from build123d import *

# Parameters (mm, degrees)
SKETCH_R        = 31.75
PAD_DEPTH       = 37.1475
SKETCH001_R     = 16.256
POCKET_DEPTH    = 19.9771
SKETCH002_R     = 16.256
POCKET001_DEPTH = 14.8463
PAD001_DEPTH    = 10.1219
SKETCH004_R     = 1.74625
POCKET002_DEPTH = 32.4241
SKETCH005_R     = 4.7879
POCKET003_DEPTH = 2.6924
SKETCH006_R     = 2.425304
POCKET004_DEPTH = 29.7317
SKETCH007_R     = 4.7879
POCKET005_DEPTH = 3.1242


with BuildPart() as part:
    # Sketch → Pad (new body)
    with BuildSketch(Plane.XY):
        Circle(SKETCH_R)
    extrude(amount=PAD_DEPTH)

    # Sketch001 → Pocket (cut)
    with BuildSketch(Plane.XY.offset(37.1475)):
        Circle(SKETCH001_R)
    extrude(amount=-POCKET_DEPTH, mode=Mode.SUBTRACT)

    # Sketch002 → Pocket001 (cut)
    with BuildSketch(Plane(origin=(0, 0, 0), x_dir=(1, 0, 0), z_dir=(0, 0, -1))):
        Circle(SKETCH002_R)
    extrude(amount=-POCKET001_DEPTH, mode=Mode.SUBTRACT)

    # Sketch003 → Pad001 (new body)
    with BuildSketch(Plane(origin=(0, 0, 14.8463), x_dir=(1, 0, 0), z_dir=(0, 0, -1))):
        with BuildLine():
            ThreePointArc((-5.67159, -3.48615), (0, -6.65734), (5.67159, -3.48615))
            Line((5.67159, -3.48615), (7.95655, -3.48615))
            ThreePointArc((7.95655, -3.48615), (11.4427, 0), (7.95655, 3.48615))
            Line((5.67159, 3.48615), (7.95655, 3.48615))
            ThreePointArc((5.67159, 3.48615), (0, 6.65734), (-5.67159, 3.48615))
            Line((-7.95655, 3.48615), (-5.67159, 3.48615))
            ThreePointArc((-7.95655, 3.48615), (-11.4427, 0), (-7.95655, -3.48615))
            Line((-7.95655, -3.48615), (-5.67159, -3.48615))
        make_face()
    extrude(amount=PAD001_DEPTH)

    # Sketch004 → Pocket002 (cut, through all)
    with BuildSketch(Plane(origin=(0, 0, 4.7244), x_dir=(1, 0, 0), z_dir=(0, 0, -1))):
        with Locations((7.95782, 0)):
            Circle(SKETCH004_R)
        with Locations((-7.95782, 0)):
            Circle(SKETCH004_R)
    extrude(amount=-POCKET002_DEPTH, mode=Mode.SUBTRACT)

    # Sketch005 → Pocket003 (cut)
    with BuildSketch(Plane(origin=(0, 0, 4.7244), x_dir=(1, 0, 0), z_dir=(0, 0, -1))):
        Circle(SKETCH005_R)
    extrude(amount=-POCKET003_DEPTH, mode=Mode.SUBTRACT)

    # Sketch006 → Pocket004 (cut, through all)
    with BuildSketch(Plane(origin=(0, 0, 7.4168), x_dir=(1, 0, 0), z_dir=(0, 0, -1))):
        Circle(SKETCH006_R)
    extrude(amount=-POCKET004_DEPTH, mode=Mode.SUBTRACT)

    # Sketch007 → Pocket005 (cut)
    with BuildSketch(Plane.XY.offset(17.1704)):
        Circle(SKETCH007_R)
    extrude(amount=-POCKET005_DEPTH, mode=Mode.SUBTRACT)


solid = part.part
Geometry check sheet. Reference: the model listing, model coordinates, mm. A direction names the side the tool comes from. Coordinates: 2 decimals unless noted, no trailing zeros. Order: outer loops, then holes, each group sorted by start corner. A loop starts at its lowest first (then second) coordinate and runs counter-clockwise, first axis right, second up. Notation, with made-up numbers: (-15, -28) - (29, -28) arc R11 cw to (29, -8) - close; hole circle Ø8 at (50, -3.75). An arc over 180 degrees is marked (long way). Answer in a Markdown table with one row per item. Add a question column.
1) Gauge pin test, flat ends, axial feed: P1, Ø1.8, axis at x = -6.5, z = 10.5, coming from the +Y side; P2, Ø15.5, axis at x = 0, y = 0, coming from the -Z side; P3, Ø2.5, axis at x = -6.5, z = 11.5, coming from the -Y side; P4, Ø2, axis at x = 23, y = -13.5, coming from the -Z side. Record the tip position at first contact, or that the pin passes through.
2) Cross-section at C-C, the plane z = 3.5. Record the cut outline in (x, y), then the cut area to 3 significant figures.
3) Release check for a two-part mould opening along X. For faces 1 (the flat face through (-8, 15, 37.148)), 2 (the cylindrical face through (4.567, 1.438, 15.63)) record: +X half, -X half, draft (parallel to the pull), parting line (faces both ways), or undercut.
4) Cross-section at A-A, the plane x = 0. Record the cut outline in (y, z), then the cut area to 3 significant figures.
5) Material ranges on line 1 along X through (y, z) = (3, 11); line 2 along Y through (x, z) = (-7, 5); line 3 along Y through (x, z) = (1.5, 14.5), recorded low to high. Write a range as [from, to].
6) Cross-section at B-B, the plane y = 0. State how many separate pieces and enclosed holes the cut face has, then the cut area to 3 significant figures.
7) Set-up check for faces 3 (the flat face through (-7, 3.486, 10)), 4 (the flat face through (3, 4, 17.17)), 5 (the flat face through (-8, 15, 0)): record each of +Z, -Z, +X, -X, +Y, -Y from which the full face is reachable in a straight line by a thin tool's end or side.
8) Cross-section at D-D, the plane y = 13. Record the cut outline in (x, z), then the cut area to 3 significant figures.
Check result:
| question | item | result |
|---|---|---|
| 1 | P1 | stops at y = 31.25 |
| 1 | P2 | stops at z = 4.72 |
| 1 | P3 | stops at y = -31.31 |
| 1 | P4 | stops at z = 0 |
| 2 | outline | circle Ø63.5 at (0, 0); hole circle Ø32.51 at (0, 0) |
| 2 | area | 2,340 mm² |
| 3 | face 1 | draft |
| 3 | face 2 | undercut |
| 4 | outline | (-31.75, 0) - (-16.26, 0) - (-16.26, 14.85) - (-6.66, 14.85) - (-6.66, 4.72) - (-4.79, 4.72) - (-4.79, 7.42) - (-2.43, 7.42) - (-2.43, 14.05) - (-4.79, 14.05) - (-4.79, 17.17) - (-16.26, 17.17) - (-16.26, 37.15) - (-31.75, 37.15) - close; (2.43, 7.42) - (4.79, 7.42) - (4.79, 4.72) - (6.66, 4.72) - (6.66, 14.85) - (16.26, 14.85) - (16.26, 0) - (31.75, 0) - (31.75, 37.15) - (16.26, 37.15) - (16.26, 17.17) - (4.79, 17.17) - (4.79, 14.05) - (2.43, 14.05) - close |
| 4 | area | 1,270 mm² |
| 5 | line 1 | x = [-31.61, -15.98], [-9.73, 9.73], [15.98, 31.61] |
| 5 | line 2 | y = [-30.97, -14.67], [-3.49, -1.46], [1.46, 3.49], [14.67, 30.97] |
| 5 | line 3 | y = [-31.71, -16.19], [-6.49, -4.55], [4.55, 6.49], [16.19, 31.71] |
| 6 | separate pieces | 4 |
| 6 | enclosed holes | 0 |
| 6 | area | 1,280 mm² |
| 7 | face 3 | -Z |
| 7 | face 4 | +Z |
| 7 | face 5 | -Z, +X, -X, +Y, -Y |
| 8 | outline | (-28.97, 0) - (-9.76, 0) - (-9.76, 14.85) - (9.76, 14.85) - (9.76, 0) - (28.97, 0) - (28.97, 37.15) - (9.76, 37.15) - (9.76, 17.17) - (-9.76, 17.17) - (-9.76, 37.15) - (-28.97, 37.15) - close |
| 8 | area | 1,470 mm² |
